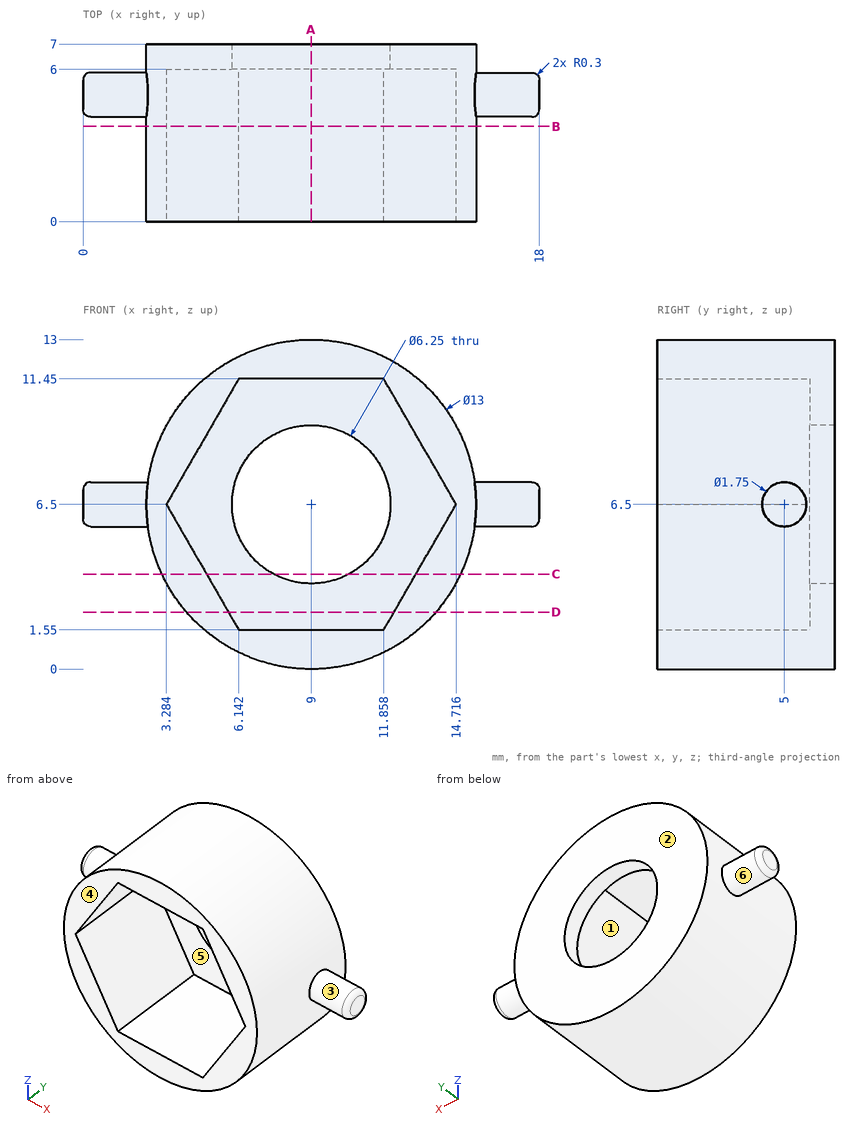
Source: three-view drawing plus pictorial views. Frame: mm from the lowest corner of the part. A direction names the side the tool comes from. Coordinates: 2 decimals unless noted, no trailing zeros. Loops run counter-clockwise (first coordinate to the right, second up) from the corner with the lowest first, then second, coordinate; pieces in that order, holes last. Notation, with made-up numbers: (60.5, 15.5) -> (111.5, 15.5) arc R19 ccw to (111.5, 33.5) -> close; hole circle Ø11 at (58, 14.5). An arc over 180 degrees is marked (long way). One line per item, written item: value.
(1) Set-up query: the marked faces 4, 5 and 6. Return all of +Z, -Z, +X, -X, +Y, -Y with unobstructed straight access to the full face (end or side cutting, diameter ignored); none if empty.
Answer below:
face 4: +Z, -Z, +X, -X, -Y
face 5: -Y
face 6: -X
(2) Ray query, line 1 along Z through (x, y) = (9, 6.4) (3 decimals); line 2 along Y through (x, z) = (10.5, 2.5); line 3 along Z through (x, y) = (13.25, 1.5). Return the intervals inside material, ascending.
Answer below:
line 1: z = 0 to 3.375, 9.625 to 13
line 2: y = 6 to 7
line 3: z = 1.58 to 3.96, 9.04 to 11.42
(3) Cut plane B-B (y = 3.75). Output: boundary loops of the cut face in (x, z).
Answer below:
outline: circle Ø13 at (9, 6.5); hole (3.28, 6.5) -> (6.14, 1.55) -> (11.86, 1.55) -> (14.72, 6.5) -> (11.86, 11.45) -> (6.14, 11.45) -> close
(4) Draft query along Z for the marked faces 1, 2 and 3. Return one class per face: pulls with the +Z half, pulls with the -Z half, needs draft (parallel to the pull), parting line crosses it, or undercut.
Answer below:
face 1: undercut
face 2: needs draft
face 3: parting line crosses it
(5) Pin query (flat end, axial travel): pin 1 Ø2 at (x, y) = (7.5, 6) entering from +Z; pin 2 Ø4 at (y, z) = (1.5, 11.5) entering from -X. Return the tip coordinate at first contact, or that it passes through.
Answer below:
pin 1: stops at z = 12.98
pin 2: stops at x = 3.23
(6) Cut plane A-A (x = 9). Output: boundary loops of the cut face in (y, z) (3 decimals).
Answer below:
outline: (0, 0) -> (7, 0) -> (7, 3.375) -> (6, 3.375) -> (6, 1.55) -> (0, 1.55) -> close; (0, 11.45) -> (6, 11.45) -> (6, 9.625) -> (7, 9.625) -> (7, 13) -> (0, 13) -> close
(7) Cut plane D-D (z = 2.25). Output: boundary loops of the cut face in (x, y).
Answer below:
outline: (4.08, 0) -> (5.74, 0) -> (5.74, 6) -> (12.26, 6) -> (12.26, 0) -> (13.92, 0) -> (13.92, 7) -> (4.08, 7) -> close
(8) Cut plane C-C (z = 3.75). Output: boundary loops of the cut face in (x, y).
Answer below:
outline: (3.11, 0) -> (4.87, 0) -> (4.87, 6) -> (7.52, 6) -> (7.52, 7) -> (3.11, 7) -> close; (10.48, 6) -> (13.13, 6) -> (13.13, 0) -> (14.89, 0) -> (14.89, 7) -> (10.48, 7) -> close
